Autodesk Inventor part; units mm, degrees
ref_plane "Arbeitsebene1" through (0, 0, 0) normal (0, 0, 1) x (1, 0, 0)
ref_plane "YZ Plane" through (0, 0, 0) normal (1, 0, 0) x (0, 1, 0)
ref_plane "XZ Plane" through (0, 0, 0) normal (0, 1, 0) x (-1, 0, 0)
sketch "Skizze1" plane through (0, 0, 0) normal (1, 0, 0) x (0, 1, 0)
  circle A0 centre (-99.913, 0) radius 13
  circle A1 centre (-99.913, 0) radius 10.95
  circle A2 centre (0, 0) radius 9
  arc A3 (-98.7442, 12.9473) -> (-0.0904, 8.9995) centre (-10, 995.9932) ccw
  arc A4 (-0.0904, -8.9995) -> (-98.7442, -12.9473) centre (-10, -995.9932) ccw
  circle A5 centre (0, 0) radius 5.1
  dimension "d0" = 26
  dimension "d1" = 99.913
  dimension "d2" = 21.9
  dimension "d3" = 18
  dimension "d6" = 0
  dimension "d7" = 0
  dimension "d8" = 0
  dimension "d9" = 10
  dimension "d10" = 10
  dimension "d11" = 10.2
extrude "Extrusion1" add sketch "Skizze1" along normal blind 10
ref_plane "Arbeitsebene1" through (0, 0, 0) normal (0, 0, 1) x (1, 0, 0)
properties part number "Hebel"
The listing builds one solid part. Answer for the finished solid, in the listing's coordinates (mm). Coordinates: 2 decimals unless noted, no trailing zeros. Write each loop counter-clockwise with the first axis right and the second up, starting at its lowest first coordinate (ties: lowest second). Pieces come first, ordered by that corner, then holes. Notation, with made-up numbers: M -28,-2.5 L 31,-2.5 A27 cw 31,28.5 Z; hole C -23,69 d7. An arc over 180 degrees is marked long. Use a Markdown table: item, result. Add a question column.
1. Section B-B (y = -3) is taken. Give the vertices of the cut face in (x, z).
2. Given P1, Ø13, axis at y = -99.913, z = 0, coming from the +X side; P2, Ø5, axis at x = 2, y = -4, coming from the +Z side, each flat-ended and moving along its own axis, determine where each tip first touches the part or whether it passes through.
3. Straight lines are drawn through the part: line 1 along Z through (x, y) = (7.5, 0); line 2 along Z through (x, y) = (6, -16.5); line 3 along Z through (x, y) = (5, -3.5). For each, find the intervals that lie inside material, in ascending order. Write a range as [from, to].
4. Section A-A (z = 0) is taken. Give the vertices of the cut face in (x, y), plus the area to 3 significant figures.
5. For a pull along Y with two mould halves and no side action, classify faces 1 (the cylindrical face through (4.9, -89.8, 4.2)), 2 (the flat face through (0, -53, 0)) as +Y half, -Y half, draft (parallel to the pull), parting line (faces both ways), or undercut.
6. Section C-C (x = 3.5) is taken. Give the vertices of the cut face in (y, z), plus the area to 3 significant figures.
7. Section D-D (y = -105) is taken. Give the vertices of the cut face in (x, z), plus the area to 3 significant figures.
Data:
| question | item | result |
|---|---|---|
| 1 | outline | M 0,-8.97 L 10,-8.97 L 10,-4.12 L 0,-4.12 Z; M 0,4.12 L 10,4.12 L 10,8.97 L 0,8.97 Z |
| 2 | P1 | passes through |
| 2 | P2 | stops at z = 8.99 |
| 3 | line 1 | z = [-9, -5.1], [5.1, 9] |
| 3 | line 2 | z = [-8.97, 8.97] |
| 3 | line 3 | z = [-8.97, -3.71], [3.71, 8.97] |
| 4 | outline | M 0,-112.91 L 10,-112.91 L 10,-110.86 L 0,-110.86 Z; M 0,-88.96 L 10,-88.96 L 10,-5.1 L 0,-5.1 Z; M 0,5.1 L 10,5.1 L 10,9 L 0,9 Z |
| 4 | area | 898 mm2 |
| 5 | face 1 | undercut |
| 5 | face 2 | draft |
| 6 | outline | M -98.74,-12.95 A987.05 cw -0.09,-9 A9 ccw long -0.09,9 A987.04 cw -98.74,12.95 A13 ccw long Z; hole C -99.91,0 d21.9; hole C 0,0 d10.2 |
| 6 | area | 1,970 mm2 |
| 7 | outline | M 0,-11.96 L 10,-11.96 L 10,-9.7 L 0,-9.7 Z; M 0,9.7 L 10,9.7 L 10,11.96 L 0,11.96 Z |
| 7 | area | 45.3 mm2 |
